Could you check a few things on this model? Use its own coordinates, in mm. Face numbers are marked on the shaded views. A direction names the side the tool comes from. Round coordinates to 2 decimals unless told otherwise and drop trailing zeros. Write each loop counter-clockwise with the first axis right and the second up, starting at its lowest first coordinate (ties: lowest second). Pieces come first, ordered by that corner, then holes. Notation, with made-up numbers: (11, 26.5) -> (27, 26.5) arc R15 ccw to (27, 44.5) -> close; hole circle Ø11 at (-18.75, 57.25). An arc over 180 degrees is marked (long way). Return JSON: item names as keys, results as strings.
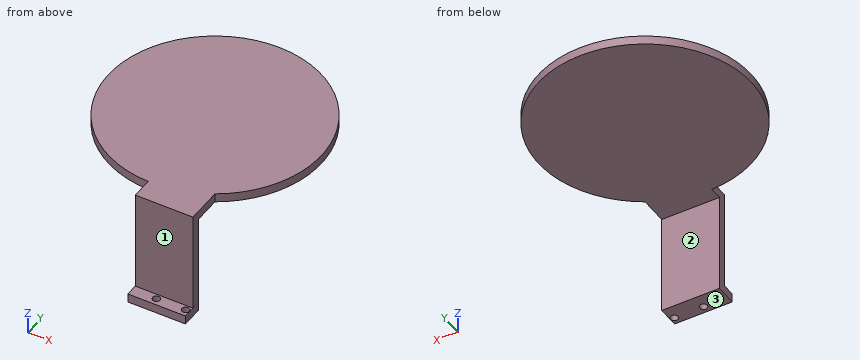
from build123d import *

# Parameters (mm, degrees)
SKETCH2_W           = 32.54
SKETCH2_H           = 8
SKETCH2_R           = 2.1
BOSS_EXTRUDE1_DEPTH = 5
SKETCH3_W           = 32.54
SKETCH3_H           = 5
BOSS_EXTRUDE2_DEPTH = 4
SKETCH4_W           = 32.539746062
SKETCH4_H           = 5
BOSS_EXTRUDE3_DEPTH = 57
SKETCH5_W           = 32.539746062
SKETCH5_H           = 5
BOSS_EXTRUDE4_DEPTH = 27.5
SKETCH7_R           = 60
BOSS_EXTRUDE6_DEPTH = 5


with BuildPart() as part:
    # Sketch2 → Boss-Extrude1 (new body)
    with BuildSketch(Plane.XY.offset(-25141.064740445)):
        with Locations((360.568878819, -3596.065695557)):
            Rectangle(SKETCH2_W, SKETCH2_H)
        with Locations((374.501060255, -3596.060789622)):
            Circle(SKETCH2_R, mode=Mode.SUBTRACT)
        with Locations((358.013502112, -3596.060789622)):
            Circle(SKETCH2_R, mode=Mode.SUBTRACT)
    extrude(amount=BOSS_EXTRUDE1_DEPTH)

    # Sketch3 → Boss-Extrude2 (add)
    with BuildSketch(Plane(origin=(0, -3592.065695557, 0), x_dir=(1, 0, 0), z_dir=(0, 1, 0))):
        with Locations((360.568878819, 25138.564740445)):
            Rectangle(SKETCH3_W, SKETCH3_H)
    extrude(amount=BOSS_EXTRUDE2_DEPTH)

    # Sketch4 → Boss-Extrude3 (add)
    with BuildSketch(Plane.XY.offset(-25136.064740445)):
        with Locations((360.56875185, -3590.565695557)):
            Rectangle(SKETCH4_W, SKETCH4_H)
    extrude(amount=BOSS_EXTRUDE3_DEPTH)

    # Sketch5 → Boss-Extrude4 (add)
    with BuildSketch(Plane(origin=(0, -3588.065695557, 0), x_dir=(1, 0, 0), z_dir=(0, 1, 0))):
        with Locations((360.56875185, 25081.564740445)):
            Rectangle(SKETCH5_W, SKETCH5_H)
    extrude(amount=BOSS_EXTRUDE4_DEPTH)

    # Sketch7 → Boss-Extrude6 (add)
    with BuildSketch(Plane.XY.offset(-25079.064740445)):
        with Locations((345.94627105, -3520.972176103)):
            Circle(SKETCH7_R)
    extrude(amount=-BOSS_EXTRUDE6_DEPTH)


solid = part.part
1) I want a section at A-A, the plane z = -25126. Please give me the cut outline in (x, y).
Return value:
{"outline": "(344.3, -3593.07) -> (376.84, -3593.07) -> (376.84, -3588.07) -> (344.3, -3588.07) -> close"}
2) I want a section at C-C, the plane y = -3497. Please give me the cut outline in (x, z).
Return value:
{"outline": "(290.94, -25084.06) -> (400.95, -25084.06) -> (400.95, -25079.06) -> (290.94, -25079.06) -> close"}
3) If I drill on probe 1 along Z at (x, y) = (356, -3558); probe 2 along Y at (x, z) = (346, -25128.5), over which ranges is the centre line in solid material (lowest first)? Write a range as [from, to].
Return value:
{"probe 1": "[-25084.06, -25079.06]", "probe 2": "[-3593.07, -3588.07]"}
4) Will these pins go through, and if not, where does the flat tip stop? pin 1 Ø2.5 at (y, z) = (-3596, -25139) entering from +X; pin 2 Ø4 at (x, y) = (358.01, -3596.06) entering from -Z; pin 3 Ø10 at (x, z) = (366.5, -25131) entering from +Y; pin 4 Ø21 at (y, z) = (-3594, -25111.5) entering from -X.
Return value:
{"pin 1": "x = 376.84", "pin 2": "through", "pin 3": "y = -3588.07", "pin 4": "x = 344.3"}
5) I want a section at B-B, the plane x = 369.5. Please give me the cut outline in (y, z).
Return value:
{"outline": "(-3600.07, -25141.06) -> (-3588.07, -25141.06) -> (-3588.07, -25084.06) -> (-3465.79, -25084.06) -> (-3465.79, -25079.06) -> (-3593.07, -25079.06) -> (-3593.07, -25136.06) -> (-3600.07, -25136.06) -> close"}
6) For the marked faces 1, 2 and 3, which set-ups out of +Z, -Z, +X, -X, +Y, -Y let a thin tool reach every point of the face, with its end or its side?
Return value:
{"face 1": "+Z, +X, -X, -Y", "face 2": "-Z, +X, -X, +Y", "face 3": "-Z, +X, -X, +Y, -Y"}
